from build123d import *

# Parameters (mm, degrees)
BOSS_EXTRUDE1_DEPTH = 10
CUT_EXTRUDE1_DEPTH  = 10
SKETCH2_3_W         = 3
SKETCH2_3_H         = 3
SKETCH2_3_W_2       = 6
SKETCH2_3_H_2       = 6
CUT_EXTRUDE2_DEPTH  = 6
CHAMFER2_SIZE       = 5
CHAMFER2_SIZE_2     = 10.028448541
CHAMFER3_SIZE2      = 4.999988835
CHAMFER3_SIZE       = 10
SKETCH1_6_W         = 6
SKETCH1_6_H         = 3
SKETCH1_6_W_2       = 10
SKETCH1_6_H_2       = 10
SKETCH1_6_H_3       = 6
CUT_EXTRUDE3_DEPTH  = 10
SKETCH1_7_W         = 5
SKETCH1_7_H         = 5
CUT_EXTRUDE4_DEPTH  = 5
SKETCH5_W           = 120
SKETCH5_H           = 5
BOSS_EXTRUDE3_DEPTH = 20
FILLET2_R           = 2.5


# Some blends are built 0.0001 mm under size
with BuildPart() as part:
    # Sketch1 → Boss-Extrude1 (new body)
    with BuildSketch(Plane(origin=(0, 0, 0), x_dir=(1, 0, 0), z_dir=(0, 1, 0))):
        Polygon((-60, 50), (-60, -2.5), (-60, -50), (0, -50), (60, -50), (60, 50), (0, 50), align=None)
    extrude(amount=-BOSS_EXTRUDE1_DEPTH)

    # Sketch2 → Cut-Extrude1 (cut)
    with BuildSketch(Plane.XZ.offset(10)):
        Polygon((45, 45), (-45, 45), (-45, 5), (-40, 5), (45, 5), (45, 25), align=None)
    extrude(amount=-CUT_EXTRUDE1_DEPTH, mode=Mode.SUBTRACT)

    # Sketch2<3> → Cut-Extrude2 (cut)
    with BuildSketch(Plane.XZ.offset(10)):
        with Locations((47.5, 47.5)):
            Rectangle(SKETCH2_3_W, SKETCH2_3_H)
        with Locations((-47.5, 2.5)):
            Rectangle(SKETCH2_3_W, SKETCH2_3_H)
        with Locations((47.5, 2.5)):
            Rectangle(SKETCH2_3_W, SKETCH2_3_H)
        with Locations((45, -25)):
            Rectangle(SKETCH2_3_W_2, SKETCH2_3_H_2)
        with Locations((-47.5, 47.5)):
            Rectangle(SKETCH2_3_W, SKETCH2_3_H)
        with Locations((-45, -25)):
            Rectangle(SKETCH2_3_W_2, SKETCH2_3_H_2)
    extrude(amount=-CUT_EXTRUDE2_DEPTH, mode=Mode.SUBTRACT)

    # Chamfer2
    # the kernel refuses this chamfer: 10.028448541, 5 mm, written as the material it takes off along each edge
    with BuildSketch(Plane(origin=(-45, 0, 45), x_dir=(-0.9976061957759285, 0.06915112543899754, 0), z_dir=(0, 0, -1))) as chamfer2_piece_1:
        Polygon((CHAMFER2_SIZE * 0.997606195776, -CHAMFER2_SIZE * 0.069151125439), (-CHAMFER2_SIZE_2 * 0.069151125441, -CHAMFER2_SIZE_2 * 0.997606195805), (0, 0), align=None)
    extrude(amount=40, mode=Mode.SUBTRACT)

    # Chamfer3
    chamfer3_edges = [part.edges().sort_by_distance(p)[0] for p in [
        (45, 0, 25),
    ]]
    chamfer3_side = [part.faces().sort_by_distance(p)[0] for p in [
        (45, -0.099999777, 25),
    ]]
    chamfer(chamfer3_edges, length=CHAMFER3_SIZE - 0.0001, length2=CHAMFER3_SIZE2 - 0.0001, reference=chamfer3_side[0])  # a hair under: the kernel refuses the full size

    # Sketch1<6> → Cut-Extrude3 (cut)
    # profile 1 of 6: a face of its own
    with BuildSketch(Plane(origin=(0, 0, 0), x_dir=(1, 0, 0), z_dir=(0, 1, 0))):
        Polygon((-50, 25), (-50, 30), (-60, 30), (-60, 25), (-58, 25), (-58, 28), (-52, 28), (-52, 25), align=None)
    # profile 2 of 6: a face of its own
    with BuildSketch(Plane(origin=(0, 0, 0), x_dir=(1, 0, 0), z_dir=(0, 1, 0))):
        with Locations((-55, 26.5)):
            Rectangle(SKETCH1_6_W, SKETCH1_6_H)
    # profile 3 of 6: a face of its own
    with BuildSketch(Plane(origin=(0, 0, 0), x_dir=(1, 0, 0), z_dir=(0, 1, 0))):
        with Locations((-55, 23.5)):
            Rectangle(SKETCH1_6_W, SKETCH1_6_H)
    # profile 4 of 6: a face of its own
    with BuildSketch(Plane(origin=(0, 0, 0), x_dir=(1, 0, 0), z_dir=(0, 1, 0))):
        Polygon((-50, 20), (-50, 25), (-52, 25), (-52, 22), (-58, 22), (-58, 25), (-60, 25), (-60, 20), (-55, 20), align=None)
    # profile 5 of 6: a face of its own
    with BuildSketch(Plane(origin=(0, 0, 0), x_dir=(1, 0, 0), z_dir=(0, 1, 0))):
        with Locations((55, 25)):
            Rectangle(SKETCH1_6_W_2, SKETCH1_6_H_2)
        with Locations((55, 25)):
            Rectangle(SKETCH1_6_W, SKETCH1_6_H_3, mode=Mode.SUBTRACT)
    # profile 6 of 6: a face of its own
    with BuildSketch(Plane(origin=(0, 0, 0), x_dir=(1, 0, 0), z_dir=(0, 1, 0))):
        with Locations((55, 25)):
            Rectangle(SKETCH1_6_W, SKETCH1_6_H_3)
    extrude(amount=-CUT_EXTRUDE3_DEPTH, mode=Mode.SUBTRACT)

    # Sketch1<7> → Cut-Extrude4 (cut)
    with BuildSketch(Plane(origin=(0, 0, 0), x_dir=(1, 0, 0), z_dir=(0, 1, 0))):
        with Locations((57.5, -2.5)):
            Rectangle(SKETCH1_7_W, SKETCH1_7_H)
        with Locations((57.5, -47.5)):
            Rectangle(SKETCH1_7_W, SKETCH1_7_H)
        with Locations((-57.5, -47.5)):
            Rectangle(SKETCH1_7_W, SKETCH1_7_H)
        Polygon((-55, -5), (-55, 0), (-60, 0), (-60, -2.5), (-60, -5), align=None)
    extrude(amount=-CUT_EXTRUDE4_DEPTH, mode=Mode.SUBTRACT)

    # Sketch5 → Boss-Extrude3 (add)
    with BuildSketch(Plane(origin=(0, 0, 0), x_dir=(1, 0, 0), z_dir=(0, 1, 0))):
        with Locations((0, -52.5)):
            Rectangle(SKETCH5_W, SKETCH5_H)
        with Locations((0, 52.5)):
            Rectangle(SKETCH5_W, SKETCH5_H)
    extrude(amount=-BOSS_EXTRUDE3_DEPTH)

    # Fillet2
    fillet2_edges = [part.edges().sort_by_distance(p)[0] for p in [
        (0, -20, 50),
        (0, -20, -50),
    ]]
    fillet(fillet2_edges, radius=FILLET2_R)


solid = part.part
Design review of the part built by this model. Coordinates are the model's own, in mm. A direction names the side the tool comes from. Round coordinates to 2 decimals unless told otherwise and drop trailing zeros. Write each loop counter-clockwise with the first axis right and the second up, starting at its lowest first coordinate (ties: lowest second). Pieces come first, ordered by that corner, then holes. Notation, with made-up numbers: (-29, 47) - (-6, 47) arc R26 cw to (-6, 69) - close; hole circle Ø7 at (51, 24). An arc over 180 degrees is marked (long way). Use a Markdown table: item, result. Add a question column.
1. We need section A-A (x = -52). State the section outline as (y, z) points, then the cut area to 3 significant figures.
2. Wall thickness on probe 1 along X at (y, z) = (-5.5, -26); probe 2 along Z at (x, y) = (4, -16.25); probe 3 along Z at (x, y) = (24.5, -5.5): over which ranges is each line inside the solid? List them lowest first.
3. We need section B-B (y = -15). State the section outline as (x, z) points, then the cut area to 3 significant figures.
4. We need section D-D (x = 2). State the section outline as (y, z) points, then the cut area to 3 significant figures.
5. Clearance check with flat-ended pins moving along their axes: pin 1 (10 mm diameter, centred on x = 43, z = 20, fed in from +Y); pin 2 (1.5 mm diameter, centred on x = -47, z = 41.5, fed in from +Y); pin 3 (3 mm diameter, centred on x = 29.5, z = -8, fed in from -Y); pin 4 (4 mm diameter, centred on y = -2.5, z = 46.5, fed in from -X). State where each tip first meets the part, or that it passes through.
6. Mouldability with a two-part tool opening along Z and no side actions: class faces 1 (the face through (48, -7, -25)), 2 (the face through (-60, -5, 18)), 3 (the face through (55, -2, 48)), 4 (the face through (-1, -10, 55)) as +Z half, -Z half, draft (parallel to the pull), parting line (faces both ways), or undercut.
7. For faces 5 (the face through (-58, -2, 50)), 6 (the face through (50, -5, -25)), 7 (the face through (-48, -7, 1)), list the 3-axis set-ups (+Z, -Z, +X, -X, +Y, -Y) from which the entire face can be reached by the end or side of a thin tool; tool diameter is ignored.
Output:
| question | item | result |
|---|---|---|
| 1 | outline | (-20, -55) - (0, -55) - (0, -30) - (-10, -30) - (-10, -50) - (-17.5, -50) arc R2.5 ccw to (-20, -52.5) - close; (-20, 52.5) arc R2.5 ccw to (-17.5, 50) - (-10, 50) - (-10, -20) - (0, -20) - (0, 55) - (-20, 55) - close |
| 1 | area | 1,100 mm2 |
| 2 | probe 1 | x = -50 to -48, -42 to 42, 48 to 50 |
| 2 | probe 2 | z = -55 to -50, 50 to 55 |
| 2 | probe 3 | z = -55 to 5, 45 to 55 |
| 3 | outline | (-60, -55) - (60, -55) - (60, -50) - (-60, -50) - close; (-60, 50) - (60, 50) - (60, 55) - (-60, 55) - close |
| 3 | area | 1,200 mm2 |
| 4 | outline | (-20, -55) - (0, -55) - (0, 5) - (-10, 5) - (-10, -50) - (-17.5, -50) arc R2.5 ccw to (-20, -52.5) - close; (-20, 52.5) arc R2.5 ccw to (-17.5, 50) - (-10, 50) - (-10, 45) - (0, 45) - (0, 55) - (-20, 55) - close |
| 4 | area | 797 mm2 |
| 5 | pin 1 | stops at y = -4 |
| 5 | pin 2 | stops at y = -4.51 |
| 5 | pin 3 | stops at y = -10 |
| 5 | pin 4 | stops at x = -60 |
| 6 | face 1 | undercut |
| 6 | face 2 | draft |
| 6 | face 3 | undercut |
| 6 | face 4 | +Z half |
| 7 | face 5 | -X, +Y |
| 7 | face 6 | +X, +Y, -Y |
| 7 | face 7 | -Y |
